CAD build for the part. Positions are in the model's coordinates, mm. Round coordinates to 2 decimals unless told otherwise and drop trailing zeros. Loops run counter-clockwise (first coordinate to the right, second up) from the corner with the lowest first, then second, coordinate; pieces in that order, holes last. Notation, with made-up numbers: M 41.5,-7.5 L 90.5,-7.5 A26 ccw 90.5,18.5 Z; hole C 49.25,79 d7. An arc over 180 degrees is marked long. Use a Markdown table: item, result. Add a question column.
(1) Band-saw the part on C-C, the plane x = 85. Write the cut outline in (y, z).
(2) Band-saw the part on B-B, the plane z = -62.5. Write the cut outline in (x, y), and give its area (3 significant figures).
(3) Band-saw the part on A-A, the plane x = 5.5. Write the cut outline in (y, z), and give its area (3 significant figures).
(4) Wall check: L1, parallel to X at y = 1.15, z = -25; L2, parallel to X at y = 0.45, z = -56; L3, parallel to X at y = 0.5, z = -13. Give the ranges that are in metal, low to high.
(5) Band-saw the part on D-D, the plane y = 1.25. Write the cut outline in (x, z), and give its area (3 significant figures).
(6) Two-plate mould, pull along X, no slides. Class faces 1 (the face through (11.352, 0.811, -26.474)), 2 (the face through (8, 1, -59)), 3 (the face through (87.1, 0.8, -7.6)): released by +X, released by -X, zero draft, split by the parting line, or undercut.
from build123d import *

# Parameters (mm, degrees)
BOSS_EXTRUDE1_DEPTH = 1.6
SKETCH2_R           = 2
CUT_EXTRUDE1_DEPTH  = 116.973315896
CUT_EXTRUDE2_REACH  = 117.973
SKETCH3_R           = 2


with BuildPart() as part:
    # Sketch1 → Boss-Extrude1 (new body)
    with BuildSketch(Plane(origin=(0, 0, 0), x_dir=(1, 0, 0), z_dir=(0, 1, 0))):
        Polygon((0, 15.5), (15.5, 0), (79.5, 0), (95, 15.5), (95, 51), (79.5, 66.5), (15.5, 66.5), (0, 51), align=None)
    extrude(amount=BOSS_EXTRUDE1_DEPTH)

    # Sketch2 → Cut-Extrude1 (cut, through all)
    with BuildSketch(Plane(origin=(0, 1.6, 0), x_dir=(1, 0, 0), z_dir=(0, 1, 0))):
        with Locations(Location((5.5, 18.5, 0), (0, 0, 270))):
            Circle(SKETCH2_R)
        with Locations(Location((77.5, 13, 0), (0, 0, 270))):
            Circle(SKETCH2_R)
        with Locations(Location((37.5, 62.5, 0), (0, 0, 270))):
            Circle(SKETCH2_R)
    extrude(amount=-CUT_EXTRUDE1_DEPTH, mode=Mode.SUBTRACT)

    # Sketch3 → Cut-Extrude2 (cut, up to next)
    with BuildSketch(Plane(origin=(0, 1.6, 0), x_dir=(1, 0, 0), z_dir=(0, 1, 0)), mode=Mode.PRIVATE) as cut_extrude2_sk1:
        with Locations(Location((10, 56, 0), (0, 0, 270))):
            Circle(SKETCH3_R)
    cut_extrude2_tool1 = extrude(cut_extrude2_sk1.sketch, amount=-CUT_EXTRUDE2_REACH, mode=Mode.PRIVATE) & part.part
    # Sketch3 → Cut-Extrude2 (cut, up to next)
    with BuildSketch(Plane(origin=(0, 1.6, 0), x_dir=(1, 0, 0), z_dir=(0, 1, 0)), mode=Mode.PRIVATE) as cut_extrude2_sk2:
        with Locations(Location((85, 56, 0), (0, 0, 270))):
            Circle(SKETCH3_R)
    cut_extrude2_tool2 = extrude(cut_extrude2_sk2.sketch, amount=-CUT_EXTRUDE2_REACH, mode=Mode.PRIVATE) & part.part
    # Sketch3 → Cut-Extrude2 (cut, up to next)
    with BuildSketch(Plane(origin=(0, 1.6, 0), x_dir=(1, 0, 0), z_dir=(0, 1, 0)), mode=Mode.PRIVATE) as cut_extrude2_sk3:
        with Locations(Location((85, 25, 0), (0, 0, 270))):
            Circle(SKETCH3_R)
    cut_extrude2_tool3 = extrude(cut_extrude2_sk3.sketch, amount=-CUT_EXTRUDE2_REACH, mode=Mode.PRIVATE) & part.part
    # Sketch3 → Cut-Extrude2 (cut, up to next)
    with BuildSketch(Plane(origin=(0, 1.6, 0), x_dir=(1, 0, 0), z_dir=(0, 1, 0)), mode=Mode.PRIVATE) as cut_extrude2_sk4:
        with Locations(Location((10, 25, 0), (0, 0, 270))):
            Circle(SKETCH3_R)
    cut_extrude2_tool4 = extrude(cut_extrude2_sk4.sketch, amount=-CUT_EXTRUDE2_REACH, mode=Mode.PRIVATE) & part.part
    add(cut_extrude2_tool1.solids().sort_by_distance((10, 1.6, -56))[0], mode=Mode.SUBTRACT)
    add(cut_extrude2_tool2.solids().sort_by_distance((85, 1.6, -56))[0], mode=Mode.SUBTRACT)
    add(cut_extrude2_tool3.solids().sort_by_distance((85, 1.6, -25))[0], mode=Mode.SUBTRACT)
    add(cut_extrude2_tool4.solids().sort_by_distance((10, 1.6, -25))[0], mode=Mode.SUBTRACT)


solid = part.part
Return value:
| question | item | result |
|---|---|---|
| 1 | outline | M 0,-61 L 1.6,-61 L 1.6,-58 L 0,-58 Z; M 0,-54 L 1.6,-54 L 1.6,-27 L 0,-27 Z; M 0,-23 L 1.6,-23 L 1.6,-5.5 L 0,-5.5 Z |
| 2 | outline | M 11.5,0 L 35.5,0 L 35.5,1.6 L 11.5,1.6 Z; M 39.5,0 L 83.5,0 L 83.5,1.6 L 39.5,1.6 Z |
| 2 | area | 109 mm^2 |
| 3 | outline | M 0,-56.5 L 1.6,-56.5 L 1.6,-20.5 L 0,-20.5 Z; M 0,-16.5 L 1.6,-16.5 L 1.6,-10 L 0,-10 Z |
| 3 | area | 68.0 mm^2 |
| 4 | L1 | 0 to 8, 12 to 83, 87 to 95 |
| 4 | L2 | 5 to 8, 12 to 83, 87 to 90 |
| 4 | L3 | 2.5 to 75.5, 79.5 to 92.5 |
| 5 | outline | M 0,-51 L 15.5,-66.5 L 79.5,-66.5 L 95,-51 L 95,-15.5 L 79.5,0 L 15.5,0 L 0,-15.5 Z; hole C 5.5,-18.5 d4; hole C 10,-56 d4; hole C 10,-25 d4; hole C 37.5,-62.5 d4; hole C 77.5,-13 d4; hole C 85,-56 d4; hole C 85,-25 d4 |
| 5 | area | 5,750 mm^2 |
| 6 | face 1 | undercut |
| 6 | face 2 | released by -X |
| 6 | face 3 | released by +X |
